Can you work these out from the model? Positions are in its coordinate system, mm. A direction names the side the tool comes from. Give positions to 0.01 mm unless a question says otherwise; leave off trailing zeros. Order: outer loops, then holes, each group sorted by start corner. A loop starts at its lowest first (then second) coordinate and runs counter-clockwise, first axis right, second up. Notation, with made-up numbers: (22.5, 43.25) -> (72.5, 43.25) arc R28 ccw to (72.5, 82.25) -> close; hole circle Ø8 at (-14, 8.5). An arc over 180 degrees is marked (long way). Answer as a JSON object with one key per item and string values.
```python
from build123d import *

# Parameters (mm, degrees)
F0_W     = 76.2
F0_H     = 15.24
F1_DEPTH = 33.02
F2_R     = 12.065
F3_DEPTH = 31.75
F4_R     = 2.9845
F5_DEPTH = 50.8
F6_R     = 5.08


with BuildPart() as f1:
    # F0 (on Right) → F1 (new body)
    with BuildSketch(Plane.YZ):
        with Locations((0, -7.62)):
            Rectangle(F0_W, F0_H)
    extrude(amount=F1_DEPTH)

    # F2 (on Right) → F3 (cut)
    with BuildSketch(Plane.YZ):
        with Locations((19.05, 0)):
            Circle(F2_R)
        with Locations((-19.05, 0)):
            Circle(F2_R)
    extrude(amount=F3_DEPTH, mode=Mode.SUBTRACT)

    # F4 (on Right) → F5 (cut)
    with BuildSketch(Plane.YZ):
        with Locations((19.05, 0)):
            Circle(F4_R)
        with Locations((-19.05, 0)):
            Circle(F4_R)
    extrude(amount=F5_DEPTH, mode=Mode.SUBTRACT)

    # F6
    f6_edges = [f1.edges().sort_by_distance(p)[0] for p in [
        (16.51, -38.1, -15.24),
        (16.51, 38.1, -15.24),
    ]]
    fillet(f6_edges, radius=F6_R)


solid = f1.part
```
1. If we section it at A-A on x = 27: Please give me the cut outline in (y, z) (3 decimals).
Worked answers:
{"outline": "(-38.1, -10.16) arc R5.08 ccw to (-33.02, -15.24) -> (33.02, -15.24) arc R5.08 ccw to (38.1, -10.16) -> (38.1, 0) -> (31.115, 0) arc R12.065 cw to (6.985, 0) -> (-6.985, 0) arc R12.065 cw to (-31.115, 0) -> (-38.1, 0) -> close"}
2. If we section it at D-D on y = -28.5: Please give me the cut outline in (x, z), then the cut area to 3 significant figures.
Worked answers:
{"outline": "(0, -15.24) -> (33.02, -15.24) -> (33.02, 0) -> (31.75, 0) -> (31.75, -7.5) -> (0, -7.5) -> close", "area": "265 mm²"}
3. For faces 5 (the face through (31.75, 19, -6)), 6 (the face through (0, -1, -9)), which set-ups out of +Z, -Z, +X, -X, +Y, -Y let a thin tool reach every point of the face, with its end or its side?
Worked answers:
{"face 5": "+Z, -X", "face 6": "+Z, -Z, -X, +Y, -Y"}
4. Please list where these lines run through material, in increasing order: L1, parallel to Y at x = 23.5, z = -3.5; L2, parallel to Y at x = 29, z = -2.25; L3, parallel to Z at x = 5.5, y = 18.5.
Worked answers:
{"L1": "-38.1 to -30.6, -7.5 to 7.5, 30.6 to 38.1", "L2": "-38.1 to -30.9, -7.2 to 7.2, 30.9 to 38.1", "L3": "-15.24 to -12.05"}
5. If we section it at C-C on z = -4.5: Please give me the cut outline in (x, y), then the cut area to 3 significant figures.
Worked answers:
{"outline": "(0, -38.1) -> (33.02, -38.1) -> (33.02, 38.1) -> (0, 38.1) -> (0, 30.24) -> (31.75, 30.24) -> (31.75, 7.86) -> (0, 7.86) -> (0, -7.86) -> (31.75, -7.86) -> (31.75, -30.24) -> (0, -30.24) -> close", "area": "1,090 mm²"}
6. Will these pins go through, and if not, where does the flat tip stop? pin 1 Ø1.5 at (x, y) = (5, 24.5) entering from +Z; pin 2 Ø3 at (x, y) = (19.5, -18) entering from +Z.
Worked answers:
{"pin 1": "z = -10.35", "pin 2": "z = -11.79"}
7. If we mould it in two halves opening along Y, with no side actions, what happens to faces 1 (the face through (16, -36, 0)), 2 (the face through (16, -38.1, -5)), 3 (the face through (16, 38.1, -5)), 4 (the face through (32.376, 18.984, -2.984))? For each: +Y half, -Y half, draft (parallel to the pull), parting line (faces both ways), or undercut.
Worked answers:
{"face 1": "draft", "face 2": "-Y half", "face 3": "+Y half", "face 4": "undercut"}
